```python
from build123d import *

# Parameters (mm, degrees)
SKETCH1_R               = 17.5
BOSS_EXTRUDE1_DEPTH     = 2
SKETCH2_R               = 1.25
CUT_EXTRUDE1_DEPTH      = 5
CIRPATTERN1_COUNT       = 6
SKETCH3_R               = 5
BOSS_EXTRUDE2_DEPTH     = 30
SKETCH4_W               = 50
SKETCH4_H               = 20
BOSS_EXTRUDE3_DEPTH     = 7
SKETCH5_W               = 7
SKETCH5_H               = 20
BOSS_EXTRUDE4_DEPTH     = 60
SKETCH6_R               = 0.875
CUT_EXTRUDE2_DEPTH      = 7
SKETCH7_W               = 12
SKETCH7_H               = 23
CUT_EXTRUDE3_DEPTH      = 7
SKETCH8_R               = 4
CUT_EXTRUDE4_DEPTH      = 32
CUT_EXTRUDE4_DEPTH_BACK = 7


with BuildPart() as part:
    # Sketch1 → Boss-Extrude1 (new body)
    with BuildSketch(Plane(origin=(0, 0, 0), x_dir=(1, 0, 0), z_dir=(0, 1, 0))):
        Circle(SKETCH1_R)
    extrude(amount=BOSS_EXTRUDE1_DEPTH)

    # Sketch2 → Cut-Extrude1 (cut)
    with BuildSketch(Plane(origin=(0, 2, 0), x_dir=(1, 0, 0), z_dir=(0, 1, 0))):
        with Locations((0, 15)):
            Circle(SKETCH2_R)
    cut_extrude1 = extrude(amount=-CUT_EXTRUDE1_DEPTH, mode=Mode.SUBTRACT)

    # CirPattern1: Cut-Extrude1 ×6 about axis
    cirpattern1_axis = Axis((0, 0, 0), (0, 1, 0))
    for i in range(1, CIRPATTERN1_COUNT):
        add(cut_extrude1.rotate(cirpattern1_axis, i * 360 / CIRPATTERN1_COUNT), mode=Mode.SUBTRACT)

    # Sketch3 → Boss-Extrude2 (add)
    with BuildSketch(Plane(origin=(0, 2, 0), x_dir=(1, 0, 0), z_dir=(0, 1, 0))):
        Circle(SKETCH3_R)
    extrude(amount=BOSS_EXTRUDE2_DEPTH)

    # Sketch4 → Boss-Extrude3 (add)
    with BuildSketch(Plane(origin=(0, 32, 0), x_dir=(1, 0, 0), z_dir=(0, 1, 0))):
        Rectangle(SKETCH4_W, SKETCH4_H)
    extrude(amount=BOSS_EXTRUDE3_DEPTH)

    # Sketch5 → Boss-Extrude4 (add)
    with BuildSketch(Plane(origin=(0, 39, 0), x_dir=(1, 0, 0), z_dir=(0, 1, 0))):
        with Locations((21.5, 0)):
            Rectangle(SKETCH5_W, SKETCH5_H)
    extrude(amount=BOSS_EXTRUDE4_DEPTH)

    # Sketch6 → Cut-Extrude2 (cut)
    with BuildSketch(Plane.ZY.offset(-18)):
        with Locations((0, 87.15)):
            Circle(SKETCH6_R)
        with Locations((0, 59)):
            Circle(SKETCH6_R)
    extrude(amount=-CUT_EXTRUDE2_DEPTH, mode=Mode.SUBTRACT)

    # Sketch7 → Cut-Extrude3 (cut)
    with BuildSketch(Plane.ZY.offset(-18)):
        with Locations((0, 73.075)):
            Rectangle(SKETCH7_W, SKETCH7_H)
    extrude(amount=-CUT_EXTRUDE3_DEPTH, mode=Mode.SUBTRACT)

    # Sketch8 → Cut-Extrude4 (cut, two sides)
    with BuildSketch(Plane(origin=(0, 32, 0), x_dir=(-1, 0, 0), z_dir=(0, -1, 0))) as cut_extrude4_sk:
        Circle(SKETCH8_R)
    extrude(amount=CUT_EXTRUDE4_DEPTH, mode=Mode.SUBTRACT)
    extrude(cut_extrude4_sk.sketch, amount=-CUT_EXTRUDE4_DEPTH_BACK, mode=Mode.SUBTRACT)


solid = part.part
```
Here's how the part is built. I have some questions about the finished solid (model axes, mm). A direction names the side the tool comes from. Give positions to 0.01 mm unless a question says otherwise; leave off trailing zeros. Write each loop counter-clockwise with the first axis right and the second up, starting at its lowest first coordinate (ties: lowest second). Pieces come first, ordered by that corner, then holes. Notation, with made-up numbers: M 32,-37 L 72,-37 A20 ccw 72,-1 Z; hole C 74.25,-12 d7. An arc over 180 degrees is marked long. Put each result on its own line as item: value. Start each with the question number.
Item 1: If we section it at C-C, the plane y = 19: Write out the boundary of the cut face in (x, z), then the cut area to 3 significant figures.
Item 2: If we section it at D-D, the plane z = -15: Write out the boundary of the cut face in (x, y).
Item 3: On a 3-axis mill with a long thin cutter (end or side, diameter ignored), from which of +Z, -Z, +X, -X, +Y, -Y can I reach the whole of each face in a straight line? I mean faces 1 (the flat face through (18, 69, 7)), 2 (the cylindrical face through (-13.662, 1.014, -6.446)), 3 (the flat face through (21, 73, 6)). Say none if no direction works.
Item 4: If we section it at B-B, the plane z = -7.5: Write out the boundary of the cut face in (x, y), then the cut area to 3 significant figures.
Item 5: Thinking about a two-plate mould opening in X: for faces 4 (the flat face through (21, 99, 0)), 5 (the cylindrical face through (-13.26, 1.01, 8.72)), 6 (the flat face through (-25, 35, 0)), which applies, +X half, -X half, draft (parallel to the pull), parting line (faces both ways), or undercut?
Item 6: I need wall thicknesses on L1, parallel to Y at x = 20.5, z = 0 (3 decimals); L2, parallel to Z at x = 20, y = 59 (3 decimals); L3, parallel to Y at x = -5, z = 1. Which ranges of each line are inside material? Lowest first, please. Write a range as from..to.
Item 7: If we section it at A-A, the plane x = 0: Write out the boundary of the cut face in (y, z), then the cut area to 3 significant figures.
Item 8: Will these pins go through, and if not, where does the flat tip stop? pin 1 (1.1 mm diameter, centred on y = 59, z = 0, fed in from +X) (3 decimals); pin 2 (1 mm diameter, centred on y = 82, z = -9.5, fed in from -X); pin 3 (2 mm diameter, centred on x = 20, z = 2.5, fed in from -Y); pin 4 (7.5 mm diameter, centred on x = 22, y = 69.5, fed in from -Z).
Values:
1. outline: C 0,0 d10; hole C 0,0 d8
1. area: 28.3 mm²
2. outline: M -9.01,0 L -1.25,0 L -1.25,2 L -9.01,2 Z; M 1.25,0 L 9.01,0 L 9.01,2 L 1.25,2 Z
3. face 1: +Z, -Z, -X, +Y
3. face 2: -Y
3. face 3: +X, -X
4. outline: M -25,32 L 25,32 L 25,99 L 18,99 L 18,39 L -25,39 Z; M -15.81,0 L -14.24,0 L -14.24,2 L -15.81,2 Z; M -11.74,0 L 11.74,0 L 11.74,2 L -11.74,2 Z; M 14.24,0 L 15.81,0 L 15.81,2 L 14.24,2 Z
4. area: 823 mm²
5. face 4: draft
5. face 5: undercut
5. face 6: -X half
6. L1: 32..58.125, 59.875..61.575, 84.575..86.275, 88.025..99
6. L2: -10..-0.875, 0.875..10
6. L3: 0..2, 32..39
7. outline: M 0,-17.5 L 2,-17.5 L 2,-16.25 L 0,-16.25 Z; M 0,-13.75 L 2,-13.75 L 2,-5 L 32,-5 L 32,-10 L 39,-10 L 39,-4 L 0,-4 Z; M 0,4 L 39,4 L 39,10 L 32,10 L 32,5 L 2,5 L 2,13.75 L 0,13.75 Z; M 0,16.25 L 2,16.25 L 2,17.5 L 0,17.5 Z
7. area: 188 mm²
8. pin 1: through
8. pin 2: x = 18
8. pin 3: y = 32
8. pin 4: z = -10
